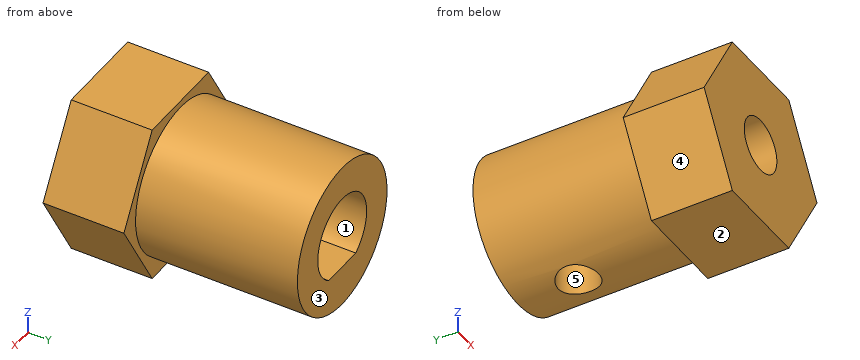
```python
from build123d import *

# Parameters (mm, degrees)
SALIENTE_EXTRUIR1_DEPTH = 6
CROQUIS_BODY_R          = 5.5
SALIENTE_EXTRUIR2_DEPTH = 12
CORTAR_EXTRUIR1_DEPTH   = 12
CROQUIS5_R              = 1.5
CORTAR_EXTRUIR2_DEPTH   = 3.5
CROQUIS6_R              = 2
CORTAR_EXTRUIR3_DEPTH   = 6


with BuildPart() as part:
    # Croquis hex-head → Saliente-Extruir1 (new body)
    with BuildSketch(Plane(origin=(0, 0, 0), x_dir=(1, 0, 0), z_dir=(0, 1, 0))):
        Polygon((6.92820323, 0), (3.464101615, 6), (-3.464101615, 6), (-6.92820323, 0), (-3.464101615, -6), (3.464101615, -6), align=None)
    extrude(amount=SALIENTE_EXTRUIR1_DEPTH)

    # Croquis body → Saliente-Extruir2 (add)
    with BuildSketch(Plane(origin=(0, 6, 0), x_dir=(1, 0, 0), z_dir=(0, 1, 0))):
        with Locations(Location((0, 0, 0), (0, 0, 270))):
            Circle(CROQUIS_BODY_R)
    extrude(amount=SALIENTE_EXTRUIR2_DEPTH)

    # Croquis inner → Cortar-Extruir1 (cut)
    with BuildSketch(Plane(origin=(0, 18, 0), x_dir=(1, 0, 0), z_dir=(0, 1, 0))):
        with BuildLine():
            Line((-1.658312395, 2.5), (1.658312395, 2.5))
            ThreePointArc((1.658312395, 2.5), (0, -3), (-1.658312395, 2.5))
        make_face()
    extrude(amount=-CORTAR_EXTRUIR1_DEPTH, mode=Mode.SUBTRACT)

    # Croquis5 → Cortar-Extruir2 (cut)
    with BuildSketch(Plane(origin=(0, 0, -6), x_dir=(-1, 0, 0), z_dir=(0, 0, -1))):
        with Locations((0, 13.5)):
            Circle(CROQUIS5_R)
    extrude(amount=-CORTAR_EXTRUIR2_DEPTH, mode=Mode.SUBTRACT)

    # Croquis6 → Cortar-Extruir3 (cut)
    with BuildSketch(Plane.XZ):
        with Locations(Location((0, 0, 0), (0, 0, 270))):
            Circle(CROQUIS6_R)
    extrude(amount=-CORTAR_EXTRUIR3_DEPTH, mode=Mode.SUBTRACT)


solid = part.part
```
Could you check a few things on this model? Use its own coordinates, in mm. Face numbers are marked on the shaded views. A direction names the side the tool comes from. Round coordinates to 2 decimals unless told otherwise and drop trailing zeros. Loops run counter-clockwise (first coordinate to the right, second up) from the corner with the lowest first, then second, coordinate; pieces in that order, holes last.
Q1. Please list where these lines run through material, in increasing order: L1, parallel to X at y = 8.75, z = 0; L2, parallel to Y at x = -3, z = 5; L3, parallel to X at y = 17, z = -2.
Q2. On a 3-axis mill with a long thin cutter (end or side, diameter ignored), from which of +Z, -Z, +X, -X, +Y, -Y can I reach the whole of each face in a straight line? I mean the marked faces 1 and 2. Say none if no direction works.
Q3. Thinking about a two-plate mould opening in X: for the marked faces 3, 4 and 5, which applies, pulls with the +X half, pulls with the -X half, needs draft (parallel to the pull), parting line crosses it, or undercut?
Q4. I want a section at D-D (z = -2.75). Write out the boundary of the cut face in (x, y).
Q5. For P1, Ø4, axis at y = 13, z = 3.5, coming from the +X side; P2, Ø4, axis at y = 14, z = -3, coming from the -X side; P3, Ø3, axis at x = -3.5, y = 14.5, coming from the +Z side, each with a flat end and sliding along its axis, tell me the tip position at first contact or that it passes through.
Q6. I want a section at B-B (y = 4). Write out the boundary of the cut face in (x, z).
Q7. I want a section at A-A (x = 0). Write out the boundary of the cut face in (y, z), and give its area (3 significant figures).
Q8. I want a section at C-C (z = -0.25). Write out the boundary of the cut face in (x, y).
Answer below:
1. L1: x = -5.5 to -3, 3 to 5.5
1. L2: y = 0 to 6
1. L3: x = -5.12 to -2.24, 2.24 to 5.12
2. face 1: +Y
2. face 2: -Z, +X, -X, +Y, -Y
3. face 3: needs draft
3. face 4: pulls with the -X half
3. face 5: undercut
4. outline: (-5.34, 0) - (5.34, 0) - (5.34, 6) - (4.76, 6) - (4.76, 18) - (-4.76, 18) - (-4.76, 6) - (-5.34, 6) - close; hole circle Ø3 at (0, 13.5)
5. P1: stops at x = 5.29
5. P2: stops at x = -5.41
5. P3: stops at z = 5.12
6. outline: (-6.93, 0) - (-3.46, -6) - (3.46, -6) - (6.93, 0) - (3.46, 6) - (-3.46, 6) - close; hole circle Ø4 at (0, 0)
7. outline: (0, -6) - (6, -6) - (6, -5.5) - (12, -5.5) - (12, -2.5) - (6, -2.5) - (6, -2) - (0, -2) - close; (0, 2) - (6, 2) - (6, 3) - (18, 3) - (18, 5.5) - (6, 5.5) - (6, 6) - (0, 6) - close; (15, -5.5) - (18, -5.5) - (18, -2.5) - (15, -2.5) - close
7. area: 105 mm2
8. outline: (-6.78, 0) - (-1.98, 0) - (-1.98, 6) - (-2.99, 6) - (-2.99, 18) - (-5.49, 18) - (-5.49, 6) - (-6.78, 6) - close; (1.98, 0) - (6.78, 0) - (6.78, 6) - (5.49, 6) - (5.49, 18) - (2.99, 18) - (2.99, 6) - (1.98, 6) - close
